```python
from build123d import *

# Parameters (mm, degrees)
F1_DEPTH = 15.875
F2_R     = 50.8
F3_R     = 25.4
F4_R     = 25.4
F5_R     = 1.5875
F6_DEPTH = 12.7


with BuildPart() as f1:
    # F0 (on Top) → F1 (new body)
    with BuildSketch(Plane.XY):
        Polygon((0, -901.7), (0, 0), (-952.5, 0), (-952.5, -381), (-431.8, -901.7), align=None)
    extrude(amount=-F1_DEPTH)

    # F2
    f2_edges = [f1.edges().sort_by_distance(p)[0] for p in [
        (0, -901.7, -7.9375),
    ]]
    fillet(f2_edges, radius=F2_R)

    # F3
    f3_edges = [f1.edges().sort_by_distance(p)[0] for p in [
        (-431.8, -901.7, -7.9375),
    ]]
    fillet(f3_edges, radius=F3_R)

    # F4
    f4_edges = [f1.edges().sort_by_distance(p)[0] for p in [
        (-952.5, -381, -7.9375),
    ]]
    fillet(f4_edges, radius=F4_R)

    # F5 (on face) → F6 (cut)
    with BuildSketch(Plane(origin=(0, 0, -15.875), x_dir=(1, 0, 0), z_dir=(0, 0, -1))):
        with Locations((-101.6, 50.8)):
            Circle(F5_R)
    extrude(amount=-F6_DEPTH, mode=Mode.SUBTRACT)


solid = f1.part
```
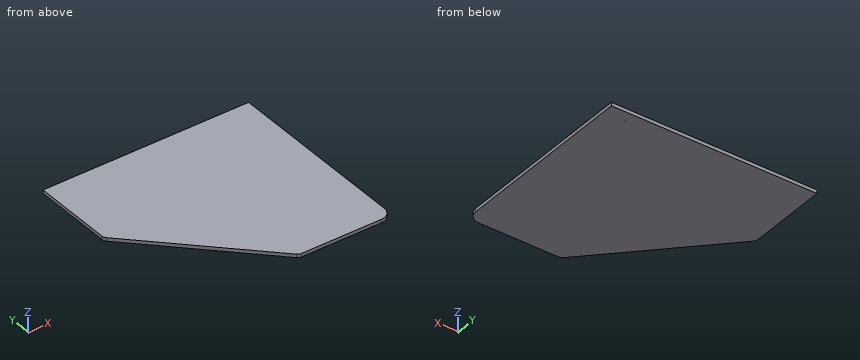
CAD build for the part. Positions are in the model's coordinates, mm. Round coordinates to 2 decimals unless told otherwise and drop trailing zeros. Order: outer loops, then holes, each group sorted by start corner. A loop starts at its lowest first (then second) coordinate and runs counter-clockwise, first axis right, second up.
Item 1: Pin check, flat tip, straight feed: pin 1 (2.5 mm diameter, centred on x = -101.6, y = -50.8, fed in from -Z) (3 decimals). Stop position of the tip, or through.
Item 2: Probe line 1 along Y through (x, z) = (-101.6, -7.5); line 2 along Y through (x, z) = (-102, -8.75); line 3 along X through (y, z) = (-50.8, -12.75). List the from-to ranges inside material, lowest first.
Item 3: Saw through at A-A on z = -12.5. Write the cut outline in (x, y) (1 decimal).
Item 4: Saw through at C-C on x = -691.5. Write the cut outline in (y, z) (3 decimals), then the cut area to 3 significant figures.
Item 5: Saw through at B-B on y = -835.5. Write the cut outline in (x, z) (3 decimals), then the cut area to 3 significant figures.
Reported:
1. pin 1: stops at z = -3.175
2. line 1: y = -901.7 to -52.39, -49.21 to 0
2. line 2: y = -901.7 to -52.34, -49.26 to 0
2. line 3: x = -952.5 to -103.19, -100.01 to 0
3. outline: (-952.5, -370.5) arc R25.4 ccw to (-945.1, -388.4) - (-439.2, -894.3) arc R25.4 ccw to (-421.3, -901.7) - (-50.8, -901.7) arc R50.8 ccw to (0, -850.9) - (0, 0) - (-952.5, 0) - close; hole circle Ø3.2 at (-101.6, -50.8)
4. outline: (-642, -15.875) - (0, -15.875) - (0, 0) - (-642, 0) - close
4. area: 10,200 mm2
5. outline: (-498, -15.875) - (0, -15.875) - (0, 0) - (-498, 0) - close
5. area: 7,910 mm2
